The drawing under review shows one solid part. Ordinate dimensions are in mm from its lowest x, y, z. A direction names the side the tool comes from. Give positions to 0.01 mm unless a question says otherwise; leave off trailing zeros. Loops run counter-clockwise (first coordinate to the right, second up) from the corner with the lowest first, then second, coordinate; pieces in that order, holes last.
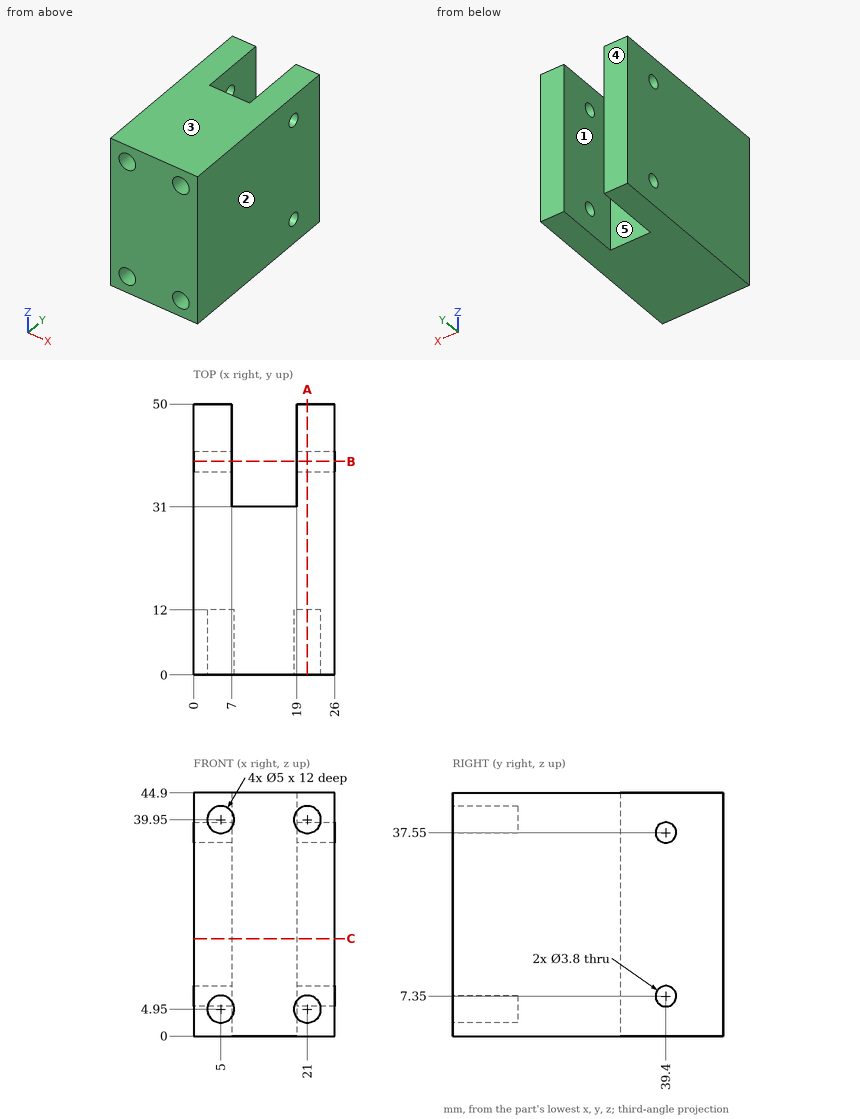
Item 1: For L1, parallel to Z at x = 5, y = 5.25; L2, parallel to X at y = 46, z = 37; L3, parallel to X at y = 3, z = 4, list the stretches that pass through material, from the lowest coordinate up.
Answer:
L1: z = 0 to 2.45, 7.45 to 37.45, 42.45 to 44.9
L2: x = 0 to 7, 19 to 26
L3: x = 0 to 2.69, 7.31 to 18.69, 23.31 to 26
Item 2: Clearance check with flat-ended pins moving along their axes: pin 1 Ø2.5 at (x, z) = (4, 5) entering from -Y; pin 2 Ø6 at (x, z) = (11.5, 12) entering from +Y. State where each tip first meets the part, or that it passes through.
Answer:
pin 1: stops at y = 12
pin 2: stops at y = 31
Item 3: Tool access review of the marked faces 4 and 5: name each direction out of +Z, -Z, +X, -X, +Y, -Y from which nothing blocks a thin tool from reaching the whole face with its end or side.
Answer:
face 4: +Z, -Z, +X, -X, +Y
face 5: +Z, -Z, +Y
Item 4: Take a section at C-C on z = 18. Give the boundary of the cut face in (x, y).
Answer:
outline: (0, 0) - (26, 0) - (26, 50) - (19, 50) - (19, 31) - (7, 31) - (7, 50) - (0, 50) - close
Item 5: Take a section at B-B on y = 39.4. Give the boundary of the cut face in (x, z).
Answer:
outline: (0, 0) - (7, 0) - (7, 5.45) - (0, 5.45) - close; (0, 9.25) - (7, 9.25) - (7, 35.65) - (0, 35.65) - close; (0, 39.45) - (7, 39.45) - (7, 44.9) - (0, 44.9) - close; (19, 0) - (26, 0) - (26, 5.45) - (19, 5.45) - close; (19, 9.25) - (26, 9.25) - (26, 35.65) - (19, 35.65) - close; (19, 39.45) - (26, 39.45) - (26, 44.9) - (19, 44.9) - close
Item 6: Take a section at A-A on x = 21. Give the boundary of the cut face in (y, z).
Answer:
outline: (0, 0) - (50, 0) - (50, 44.9) - (0, 44.9) - (0, 42.45) - (12, 42.45) - (12, 37.45) - (0, 37.45) - (0, 7.45) - (12, 7.45) - (12, 2.45) - (0, 2.45) - close; hole circle Ø3.8 at (39.4, 7.35); hole circle Ø3.8 at (39.4, 37.55)
Item 7: The part is to be moulded in two halves that separate along X. For the marked faces 1, 2 and 3, say which applies: released by +X, released by -X, zero draft, split by the parting line, or undercut.
Answer:
face 1: undercut
face 2: released by +X
face 3: zero draft
